Can you work these out from the model? Positions are in its coordinate system, mm. A direction names the side the tool comes from. Round coordinates to 2 decimals unless told otherwise and drop trailing zeros. Loops run counter-clockwise (first coordinate to the right, second up) from the corner with the lowest first, then second, coordinate; pieces in that order, holes last.
from build123d import *

# Parameters (mm, degrees)
SKETCH1_W           = 152.4
SKETCH1_H           = 50.8
BOSS_EXTRUDE1_DEPTH = 12.7
CUT_EXTRUDE1_DEPTH  = 0.95
CUT_EXTRUDE2_DEPTH  = 2
LPATTERN1_COUNT     = 2
LPATTERN1_PITCH     = 38.1
LPATTERN1_COL_COUNT = 2
LPATTERN1_COL_PITCH = 38.1


with BuildPart() as part:
    # Sketch1 → Boss-Extrude1 (new body)
    with BuildSketch(Plane(origin=(0, 0, 0), x_dir=(1, 0, 0), z_dir=(0, 1, 0))):
        with Locations((76.2, 25.4)):
            Rectangle(SKETCH1_W, SKETCH1_H)
    extrude(amount=BOSS_EXTRUDE1_DEPTH)

    # Sketch2 → Cut-Extrude1 (cut)
    with BuildSketch(Plane(origin=(0, 12.7, 0), x_dir=(1, 0, 0), z_dir=(0, 1, 0))):
        with BuildLine():
            Line((64.626998, 30.75), (64.626998, 6.35))
            Line((64.626998, 6.35), (87.773002, 6.35))
            Line((87.773002, 6.35), (87.773002, 30.75))
            ThreePointArc((87.773002, 30.75), (76.2, 42.323002), (64.626998, 30.75))
        make_face()
    cut_extrude1 = extrude(amount=-CUT_EXTRUDE1_DEPTH, mode=Mode.SUBTRACT)

    # Sketch3 → Cut-Extrude2 (cut)
    with BuildSketch(Plane(origin=(0, 11.75, 0), x_dir=(1, 0, 0), z_dir=(0, 1, 0))):
        with BuildLine():
            Line((65.626998, 30.75), (65.626998, 7.35))
            Line((65.626998, 7.35), (86.773002, 7.35))
            Line((86.773002, 7.35), (86.773002, 30.75))
            ThreePointArc((86.773002, 30.75), (76.2, 41.323002), (65.626998, 30.75))
        make_face()
    cut_extrude2 = extrude(amount=-CUT_EXTRUDE2_DEPTH, mode=Mode.SUBTRACT)

    # LPattern1: Cut-Extrude1, Cut-Extrude2 ×2
    with Locations(*[(i * LPATTERN1_PITCH, 0, 0) for i in range(1, LPATTERN1_COUNT)]):
        add(cut_extrude1, mode=Mode.SUBTRACT)
        add(cut_extrude2, mode=Mode.SUBTRACT)

    # LPattern1 col: Cut-Extrude1, Cut-Extrude2 ×2
    with Locations(*[(-i * LPATTERN1_COL_PITCH, 0, 0) for i in range(1, LPATTERN1_COL_COUNT)]):
        add(cut_extrude1, mode=Mode.SUBTRACT)
        add(cut_extrude2, mode=Mode.SUBTRACT)


solid = part.part
(1) If we section it at A-A, the plane x = 76.2: List the corners of the cut face in (y, z) for me.
Worked answers:
outline: (0, -50.8) - (12.7, -50.8) - (12.7, -42.32) - (11.75, -42.32) - (11.75, -41.32) - (9.75, -41.32) - (9.75, -7.35) - (11.75, -7.35) - (11.75, -6.35) - (12.7, -6.35) - (12.7, 0) - (0, 0) - close
(2) If we section it at B-B, the plane z = -24.5: List the corners of the cut face in (x, y) for me.
Worked answers:
outline: (0, 0) - (152.4, 0) - (152.4, 12.7) - (125.87, 12.7) - (125.87, 11.75) - (124.87, 11.75) - (124.87, 9.75) - (103.73, 9.75) - (103.73, 11.75) - (102.73, 11.75) - (102.73, 12.7) - (87.77, 12.7) - (87.77, 11.75) - (86.77, 11.75) - (86.77, 9.75) - (65.63, 9.75) - (65.63, 11.75) - (64.63, 11.75) - (64.63, 12.7) - (49.67, 12.7) - (49.67, 11.75) - (48.67, 11.75) - (48.67, 9.75) - (27.53, 9.75) - (27.53, 11.75) - (26.53, 11.75) - (26.53, 12.7) - (0, 12.7) - close
(3) Will this pin go through, and if not, where does the flat tip stop? P1, Ø11.5, axis at x = 42, z = -25, coming from the +Y side.
Worked answers:
P1: stops at y = 9.75
(4) For faces 4 (the flat face through (65, 11.75, -22)), 5 (the flat face through (0, 6, -25)), which set-ups out of +Z, -Z, +X, -X, +Y, -Y let a thin tool reach every point of the face, with its end or its side?
Worked answers:
face 4: +Y
face 5: +Z, -Z, -X, +Y, -Y
(5) If I drill on line 1 (X direction, y = 10.75, z = -29.5); line 2 (Y direction, x = 81.5, z = -18); line 3 (Z direction, x = 36.5, y = 10.75), over which ranges is the centre line in solid material (lowest first)?
Worked answers:
line 1: x = 0 to 27.53, 48.67 to 65.63, 86.77 to 103.73, 124.87 to 152.4
line 2: y = 0 to 9.75
line 3: z = -50.8 to -41.2, -7.35 to 0
(6) If we section it at C-C, the plane z = -38: List the corners of the cut face in (x, y) for me.
Worked answers:
outline: (0, 0) - (152.4, 0) - (152.4, 12.7) - (123.32, 12.7) - (123.32, 11.75) - (122, 11.75) - (122, 9.75) - (106.6, 9.75) - (106.6, 11.75) - (105.28, 11.75) - (105.28, 12.7) - (85.22, 12.7) - (85.22, 11.75) - (83.9, 11.75) - (83.9, 9.75) - (68.5, 9.75) - (68.5, 11.75) - (67.18, 11.75) - (67.18, 12.7) - (47.12, 12.7) - (47.12, 11.75) - (45.8, 11.75) - (45.8, 9.75) - (30.4, 9.75) - (30.4, 11.75) - (29.08, 11.75) - (29.08, 12.7) - (0, 12.7) - close
(7) If we mould it in two halves opening along Z, with no side actions, what happens to faces 1 (the flat face through (75, 6, 0)), 2 (the flat face through (75, 0, -26)), 3 (the cylindrical face through (114.53, 10.76, -41.32))? For each: released by +Z, released by -Z, zero draft, split by the parting line, or undercut.
Worked answers:
face 1: released by +Z
face 2: zero draft
face 3: undercut
